Source: CAD feature listing. Evaluate the final solid. Frame: model axes, mm. A direction names the side the tool comes from. Give positions to 0.01 mm unless a question says otherwise; leave off trailing zeros. Write each loop counter-clockwise with the first axis right and the second up, starting at its lowest first coordinate (ties: lowest second). Pieces come first, ordered by that corner, then holes. Notation, with made-up numbers: M 45.5,-6.5 L 89.5,-6.5 A20 ccw 89.5,17.5 Z; hole C 72.5,-36 d8. An arc over 180 degrees is marked long. Answer as a JSON object with one key per item and string values. Group by question number.
```python
from build123d import *
from OCP.BRepAlgoAPI import BRepAlgoAPI_Cut
from OCP.TopTools import TopTools_ListOfShape

# Parameters (mm, degrees)
BOSS_EXTRUDE1_DEPTH      = 1885.953741
BOSS_EXTRUDE1_DEPTH_BACK = 82.476716
SKETCH1_R                = 72


with BuildPart() as part:
    # Sketch1 → Boss-Extrude1 (new, two sides: drawn at the far end of the back side and taken through both)
    with BuildSketch(Plane.XY.offset(-BOSS_EXTRUDE1_DEPTH_BACK)):
        with Locations(Location((0, 0, 0), (0, 0, 270))):
            Circle(SKETCH1_R)
    extrude(amount=BOSS_EXTRUDE1_DEPTH + BOSS_EXTRUDE1_DEPTH_BACK)


with BuildPart() as cavity3_tool:
    # Cavity3: read off the stored shape, not the designer's step
    # Cavity3 outline → Cavity3 (revolve)
    with BuildSketch(Plane.XZ):
        with BuildLine():
            Line((72, -82.476716089), (72, 10))
            Line((72, 10), (70, 10))
            Line((70, 10), (70, -9.999999977))
            ThreePointArc((70, -9.999999977), (52.371990052, -56.445394367), (8.366438321, -79.498220911))
            ThreePointArc((8.366438321, -79.498220911), (6.48048614, -80.486199187), (5.725, -82.476716089))
            Line((5.725, -82.476716089), (72, -82.476716089))
        make_face()
        with BuildLine():
            Line((70, 1813.99999993), (70, 1794))
            Line((70, 1794), (72, 1794))
            Line((72, 1794), (72, 1885.953740521))
            Line((72, 1885.953740521), (9.315, 1885.953740521))
            ThreePointArc((9.315, 1885.953740521), (10.021717672, 1884.019611217), (11.80890411, 1882.996737486))
            ThreePointArc((11.80890411, 1882.996737486), (53.509920985, 1859.129683759), (70, 1813.99999993))
        make_face()
    revolve(axis=Axis((0, 0, 0), (0, 0, 1)))


with BuildPart() as part_1:
    add(part.part)

    # Cavity3: cut by cavity3_tool, with a tolerance
    cavity3_stock = TopTools_ListOfShape()
    cavity3_stock.Append(part_1.part.wrapped)
    cavity3_tools = TopTools_ListOfShape()
    cavity3_tools.Append(cavity3_tool.part.wrapped)
    cavity3_cut = BRepAlgoAPI_Cut()
    cavity3_cut.SetArguments(cavity3_stock)
    cavity3_cut.SetTools(cavity3_tools)
    cavity3_cut.SetFuzzyValue(0.00001)
    cavity3_cut.Build()
    add(Compound.cast(cavity3_cut.Shape()).solids(), mode=Mode.REPLACE)


solid = part_1.part
```
(1) Section B-B, the plane x = -34.5. Return loops of the section in (y, z).
(2) Ray query, L1, parallel to Y at x = -6, z = 469.5; L2, parallel to X at y = -5, z = 1587.5; L3, parallel to Z at x = -7, y = 3.5. Return the intervals inside material, ascending. Write a range as [from, to].
(3) Contact query for flat-ended pins moving along their axis: pin 1 Ø6 at (y, z) = (26, 1659) entering from +X; pin 2 Ø12 at (y, z) = (52, 604.5) entering from +X; pin 3 Ø8 at (y, z) = (8, 1374.5) entering from -X. Output: stop coordinate, or through.
(4) Access query for faces 3 (the cylindrical face through (-55.55, -42.594, 1803.86)), 4 (the flat face through (-59, 38, 10)), 5 (the cylindrical face through (21.627, -68.675, 889.512)). Directions: +Z, -Z, +X, -X, +Y, -Y. A direction counts if a zero-diameter tool reaches every point of the face in a straight line with its end or side. Return the directions, or none.
(5) Section C-C, the plane z = 1576.5. Return loops of the section in (x, y), plus the area to 3 significant figures.
(6) Pull-direction query (X, two-part tool) for faces 1 (the flat face through (59, 38, 1794)), 2 (the cylindrical face through (-55.55, -42.594, -0.14)); classes: pulls with the +X half, pulls with the -X half, needs draft (parallel to the pull), parting line crosses it, or undercut.
(7) Section A-A, the plane y = 47.5. Return loops of the section in (x, z), plus the area to 3 significant figures.
Reported:
{
 "1": {"outline": "M -63.2,10 L -60.91,10 L -60.91,-10 A60.91 ccw 60.91,-10 L 60.91,10 L 63.2,10 L 63.2,1794 L 60.91,1794 L 60.91,1814 A60.91 ccw -60.91,1814 L -60.91,1794 L -63.2,1794 Z"},
 "2": {"L1": "y = [-71.75, 71.75]", "L2": "x = [-71.83, 71.83]", "L3": "z = [-79.61, 1885.95]"},
 "3": {"pin 1": "stops at x = 68.23", "pin 2": "stops at x = 55.39", "pin 3": "stops at x = -71.89"},
 "4": {"face 3": "+Z", "face 4": "-Z", "face 5": "+Z, -Z"},
 "5": {"outline": "C 0,0 d144", "area": "16,300 mm2"},
 "6": {"face 1": "needs draft", "face 2": "parting line crosses it"},
 "7": {"outline": "M -54.11,10 L -51.42,10 L -51.42,-10 A51.42 ccw 51.42,-10 L 51.42,10 L 54.11,10 L 54.11,1794 L 51.42,1794 L 51.42,1814 A51.42 ccw -51.42,1814 L -51.42,1794 L -54.11,1794 Z", "area": "205,000 mm2"}
}
